Source: CAD feature listing. Evaluate the final solid. Frame: model axes, mm. A direction names the side the tool comes from. Round coordinates to 2 decimals unless told otherwise and drop trailing zeros. Answer as CSV lines item,"result". Start each with the question number.
Item 1: Pull-direction query (Z, two-part tool) for faces 1 (the face through (23, 19, 58)), 2 (the face through (10.02, 42.26, 32.58)), 3 (the face through (60, 13, -2)), 4 (the face through (22.913, 52.315, -31.441)); classes: +Z half, -Z half, draft (parallel to the pull), parting line (faces both ways), or undercut.
Item 2: First-contact query: P1, Ø10, axis at x = 13, z = 15.5, coming from the -Y side; P2, Ø5, axis at x = 52.5, z = -29, coming from the +Y side; P3, Ø4, axis at x = 40.5, z = 24.5, coming from the +Y side; P4, Ø10, axis at y = 27.5, z = -40, coming from the -X side. Flat tips, straight axial feed; report the tip coordinate or a pass-through.
Item 3: Set-up query: faces 5 (the face through (22.913, -60.776, 5.629)), 6 (the face through (10.02, 0.88, 53.35)), 7 (the face through (27, 40, -30)). Return all of +Z, -Z, +X, -X, +Y, -Y with unobstructed straight access to the full face (end or side cutting, diameter ignored); none if empty.
Item 4: Line query: line 1 (Y direction, x = 49, z = 0); line 2 (X direction, y = -1, z = -45.5); line 3 (Z direction, x = 39, y = 0). Output: solid intervals per line, ascending. Write a range as [from, to].
Item 5: Section query A-A on z = -5. State how many separate pieces and enclosed holes the cut face has, plus the area to 3 significant figures.
from build123d import *

# Parameters (mm, degrees)
F1_DEPTH  = 60
F2_R      = 50
F3_DEPTH  = 55
F4_R      = 12.5
F5_DEPTH  = 60.001
F8_R      = 20
F9_DEPTH  = 25
F10_COUNT = 7


with BuildPart() as f1:
    # F0 (on Right) → F1 (new body)
    with BuildSketch(Plane.YZ):
        Polygon((27.9313278908, 58), (-27.9313278908, 58), (-62.7611240755, 14.3248170156), (-50.3305137376, -40.1372453545), (0, -64.3751433221), (50.3305137376, -40.1372453545), (62.7611240755, 14.3248170156), align=None)
    extrude(amount=F1_DEPTH)

    # F2 (on face) → F3 (cut)
    with BuildSketch(Plane(origin=(0, 0, 0), x_dir=(0, -1, 0), z_dir=(-1, 0, 0))):
        Circle(F2_R)
    extrude(amount=-F3_DEPTH, mode=Mode.SUBTRACT)

    # F4 (on face) → F5 (cut, through all)
    with BuildSketch(Plane(origin=(0, 0, 0), x_dir=(0, -1, 0), z_dir=(-1, 0, 0))):
        Circle(F4_R)
    extrude(amount=-F5_DEPTH, mode=Mode.SUBTRACT)

    # F6 (on Front) → F7 (revolve)
    with BuildSketch(Plane.XZ):
        with BuildLine():
            Line((43, 17.5), (43, 12.5))
            Line((43, 12.5), (55, 12.5))
            Line((55, 12.5), (55, 22.5))
            ThreePointArc((55, 22.5), (53.5355339059, 18.9644660941), (50, 17.5))
            Line((50, 17.5), (43, 17.5))
        make_face()
    revolve(axis=Axis((55, 0, 0), (-1, 0, 0)))

    # F8 (on face) → F9 (cut)
    with BuildSketch(Plane.XY.offset(58)):
        with Locations((30, 0)):
            Circle(F8_R)
    f9 = extrude(amount=-F9_DEPTH, mode=Mode.SUBTRACT)

    # F10: F9 ×7 about axis
    f10_axis = Axis((60, 0, 0), (-1, 0, 0))
    for i in range(1, F10_COUNT):
        add(f9.rotate(f10_axis, i * 360 / F10_COUNT), mode=Mode.SUBTRACT)


solid = f1.part
Results:
1,face 1,"+Z half"
1,face 2,"undercut"
1,face 3,"draft"
1,face 4,"-Z half"
2,P1,"y = -62.76"
2,P2,"y = 53.44"
2,P3,"y = 56.24"
2,P4,"x = 0"
3,face 5,"-Z, +X, -X, -Y"
3,face 6,"+Z"
3,face 7,"-X"
4,line 1,"[-59.49, -50], [-17.5, -12.5], [12.5, 17.5], [50, 59.49]"
4,line 2,"[55, 60]"
4,line 3,"[-64.38, -50]"
5,separate pieces,"4"
5,enclosed holes,"0"
5,area,"911 mm^2"
